```python
from build123d import *

# Parameters (mm, degrees)
F3_W     = 5.571197
F3_H     = 3.305577
F4_DEPTH = 2.35


with BuildPart() as f1:
    # F0 (on Front) → F1 (revolve)
    with BuildSketch(Plane.XZ):
        with BuildLine():
            Line((0, 1), (0, 0))
            Line((0, 0), (9.673832, 0))
            Line((9.673832, 0), (19.347663, 0))
            Line((19.347663, 0), (19.347663, 1))
            Line((19.347663, 1), (17.347663, 1))
            ThreePointArc((17.347663, 1), (16.065773, 0.422657), (14.673832, 0.225))
            Line((14.673832, 0.225), (9.673832, 0.225))
            Line((9.673832, 0.225), (4.673832, 0.225))
            ThreePointArc((4.673832, 0.225), (3.28189, 0.422657), (2, 1))
            Line((2, 1), (0, 1))
        make_face()
    revolve(axis=Axis((3.460914, 0, 0), (-1, 0, 0)))

    # F3 (on offset) → F4 (cut)
    with BuildSketch(Plane.XY.offset(2.6)):
        with Locations((2.198237, 0.098479)):
            Rectangle(F3_W, F3_H)
    extrude(amount=-F4_DEPTH, mode=Mode.SUBTRACT)


solid = f1.part
```
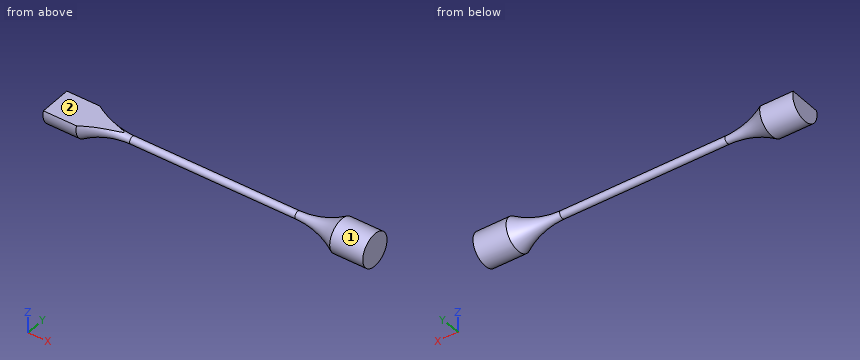
The model under review builds one solid part; all positions refer to its coordinate system, in mm. Face numbers are marked on the shaded views. A direction names the side the tool comes from. Round coordinates to 2 decimals unless told otherwise and drop trailing zeros. Loops run counter-clockwise (first coordinate to the right, second up) from the corner with the lowest first, then second, coordinate; pieces in that order, holes last. Notation, with made-up numbers: M 53.25,59.5 L 100.25,59.5 A9 ccw 100.25,71.5 Z; hole C 41.25,2.25 d1. An arc over 180 degrees is marked long. Write item = value, one per line.
Item 1: Take a section at C-C on x = 14. Write out the cut boundary in (y, z) (3 decimals), then the cut area to 3 significant figures.
Return value:
outline = C 0,0 d0.45
area = 0.159 mm2
Item 2: For line 1 (X direction, y = 0.4, z = -0.7); line 2 (X direction, y = -0.75, z = -0.6); line 3 (Y direction, x = 18.25, z = 0.25), list the stretches that pass through material, from the lowest coordinate up. Write a range as [from, to].
Return value:
line_1 = [0, 2.33], [17.01, 19.35]
line_2 = [0, 2.06], [17.28, 19.35]
line_3 = [-0.97, 0.97]
Item 3: Machinability: for the marked faces 1 and 2, which of the approach directions +Z, -Z, +X, -X, +Y, -Y give a long, thin tool a straight path to every point of the face, cutting with its end or side? Answer none if there is none.
Return value:
face_1 = +X, -X
face_2 = +Z, -X, +Y, -Y
Item 4: Insertion check: P1, Ø0.6, axis at x = 2, y = -0.5, coming from the +Z side. The pin has a flat end and moves straight along its axis. Give the tip position at first contact, or say it passes through.
Return value:
P1 = 0.25
Item 5: Take a section at B-B on z = 0. Write out the cut boundary in (x, y) (3 decimals), then the cut area to 3 significant figures.
Return value:
outline = M 0,-1 L 2,-1 A5 cw 4.674,-0.225 L 14.674,-0.225 A5 cw 17.348,-1 L 19.348,-1 L 19.348,1 L 17.348,1 A5 cw 14.674,0.225 L 4.674,0.225 A5 cw 2,1 L 0,1 Z
area = 17.6 mm2
Item 6: Take a section at A-A on y = 0. Write out the cut boundary in (x, z) (3 decimals).
Return value:
outline = M 0,-1 L 2,-1 A5 cw 4.674,-0.225 L 14.674,-0.225 A5 cw 17.348,-1 L 19.348,-1 L 19.348,1 L 17.348,1 A5 cw 14.674,0.225 L 4.674,0.225 A5 cw 4.174,0.25 L 0,0.25 Z
